```python
from build123d import *

# Parameters (mm, degrees)
SKETCH_1_R      = 3
EXTRUDE_1_DEPTH = 1
SKETCH_2_W      = 3.6
SKETCH_2_H      = 1.8
EXTRUDE_2_DEPTH = 1.8
EXTRUDE_3_DEPTH = 2
CHAMFER_1_SIZE  = 1


with BuildPart() as part:
    # 草图1 → 凸台-拉伸1 (new body)
    with BuildSketch(Plane(origin=(0, 0, 0), x_dir=(1, 0, 0), z_dir=(0, 1, 0))):
        with Locations(Location((0, 0, 0), (0, 0, 270))):
            Circle(SKETCH_1_R)
    extrude(amount=EXTRUDE_1_DEPTH)

    # 草图2 → 凸台-拉伸2 (add)
    with BuildSketch(Plane(origin=(0, 1, 0), x_dir=(1, 0, 0), z_dir=(0, 1, 0))):
        Rectangle(SKETCH_2_W, SKETCH_2_H)
    extrude(amount=EXTRUDE_2_DEPTH)

    # 草图3 → 凸台-拉伸3 (add)
    with BuildSketch(Plane(origin=(0, 2.8, 0), x_dir=(1, 0, 0), z_dir=(0, 1, 0))):
        with BuildLine():
            Line((2, 5), (-2.01, 5))
            ThreePointArc((-2.01, 5), (-5.538462838, 3.538462838), (-7, 0.01))
            Line((-7, 0.01), (-7, -0.01))
            ThreePointArc((-7, -0.01), (-5.538462838, -3.538462838), (-2.01, -5))
            Line((-2.01, -5), (2, -5))
            ThreePointArc((2, -5), (2.707106781, -4.707106781), (3, -4))
            Line((3, -4), (3, 4))
            ThreePointArc((3, 4), (2.707106781, 4.707106781), (2, 5))
        make_face()
    extrude(amount=EXTRUDE_3_DEPTH)

    # 倒角1
    chamfer_1_edges = [part.edges().sort_by_distance(p)[0] for p in [
        (-5.538462838, 4.8, 3.538462838),
        (-0.005, 4.8, 5),
        (2.707106781, 4.8, 4.707106781),
        (3, 4.8, 0),
        (2.707106781, 4.8, -4.707106781),
        (-0.005, 4.8, -5),
        (-5.538462838, 4.8, -3.538462838),
        (-7, 4.8, 0),
    ]]
    chamfer(chamfer_1_edges, length=CHAMFER_1_SIZE - 0.0001)  # a hair under: the kernel refuses the full size


solid = part.part
```
Work out the finished part from the listing and answer in its coordinate system (mm). A direction names the side the tool comes from. Round coordinates to 2 decimals unless told otherwise and drop trailing zeros. Loops run counter-clockwise (first coordinate to the right, second up) from the corner with the lowest first, then second, coordinate; pieces in that order, holes last. Notation, with made-up numbers: M 2,61.5 L 46,61.5 A23 ccw 46,98.5 Z; hole C 22.5,76.25 d3. An arc over 180 degrees is marked long. One line per question, with ' | ' between items.
Q1. Find section C-C, the plane x = -1. Give the vertices of the cut face in (y, z), then the cut area to 3 significant figures.
Conclusion:
outline: M 0,-2.83 L 1,-2.83 L 1,-0.9 L 2.8,-0.9 L 2.8,-5 L 3.8,-5 L 4.8,-4 L 4.8,4 L 3.8,5 L 2.8,5 L 2.8,0.9 L 1,0.9 L 1,2.83 L 0,2.83 Z | area: 27.9 mm2
Q2. Find section B-B, the plane x = 0. Give the vertices of the cut face in (y, z).
Conclusion:
outline: M 0,-3 L 1,-3 L 1,-0.9 L 2.8,-0.9 L 2.8,-5 L 3.8,-5 L 4.8,-4 L 4.8,4 L 3.8,5 L 2.8,5 L 2.8,0.9 L 1,0.9 L 1,3 L 0,3 Z
Q3. Find section D-D, the plane y = 0.5. Give the vertices of the cut face in (x, z).
Conclusion:
outline: C 0,0 d6
Q4. Each of these flat-tipped pins is pushed along its axis until it touches: pin 1 Ø1.4 at (y, z) = (2, 0) entering from -X; pin 2 Ø0.5 at (x, y) = (0, 1.5) entering from -Z; pin 3 Ø0.5 at (x, y) = (0.5, 2.5) entering from +Z. Where does it stop, or does it pass through?
Conclusion:
pin 1: stops at x = -1.8 | pin 2: stops at z = -0.9 | pin 3: stops at z = 0.9
Q5. The mould has two halves that part along Y. Classify faces 1 (the flat face through (0, 0, 0)), 2 (the conical face through (2.362, 4.293, -4.355)), 3 (the flat face through (0, 1, 1.3)): +Y half, -Y half, draft (parallel to the pull), parting line (faces both ways), or undercut.
Conclusion:
face 1: -Y half | face 2: +Y half | face 3: undercut
Q6. Consider line 1 along Y through (x, z) = (1, 2.25); line 2 along Y through (x, z) = (-3.75, -1.25); line 3 along Z through (x, y) = (-1.5, 1.45). Determine where each line is inside the solid, lowest interval first. Write a range as from..to.
Conclusion:
line 1: y = 0..1, 2.8..4.8 | line 2: y = 2.8..4.8 | line 3: z = -0.9..0.9
Q7. A tool of negligible diameter and unlimited length cuts with its end or side. For faces 4 (the flat face through (1.8, 2, 0)), 5 (the flat face through (0, 2, 0.9)), 6 (the flat face through (0, 2, -0.9)), 7 (the cylindrical face through (0.9, 0.49, 2.86)), from which of +Z, -Z, +X, -X, +Y, -Y can it reach the whole face along a straight path? Write none if from no direction.
Conclusion:
face 4: +Z, -Z, +X | face 5: +Z, +X, -X | face 6: -Z, +X, -X | face 7: -Y
